Autodesk Inventor part; units mm, degrees
ref_plane "YZ Plane" through (0, 0, 0) normal (1, 0, 0) x (0, 1, 0)
ref_plane "XZ Plane" through (0, 0, 0) normal (0, 1, 0) x (-1, 0, 0)
ref_plane "XY Plane" through (0, 0, 0) normal (0, 0, 1) x (1, 0, 0)
sketch "Эскиз1" plane through (0, 0, 0) normal (0, 0, 1) x (1, 0, 0)
  line L0 (50, -27) -> (-50, -27)
  line L1 (-50, -27) -> (-50, 27)
  line L2 (-50, 27) -> (50, 27)
  line L3 (50, 27) -> (50, -27)
  line L4 (50, -27) -> (-50, 27) construction
  line L5 (-50, -27) -> (50, 27) construction
  circle A0 centre (27.5, 0) radius 16.1
  point P0 (0, 0)
  point P1 (0, 0)
  dimension "d0" = 100
  dimension "d1" = 54
  dimension "d2" = 32.2
  dimension "d3" = 22.5
extrude "Выдавливание1" add sketch "Эскиз1" along normal blind 10
sketch "Эскиз2" plane through (0, 0, 0) normal (0, 0, -1) x (-1, 0, 0)
  circle A0 centre (-27.5, 0) radius 16.1
  circle A1 centre (-27.5, 0) radius 14
  point P0 (0, 0)
  dimension "d6" = 28
extrude "Выдавливание2" add sketch "Эскиз2" against normal blind 3
sketch "Эскиз3" plane through (0, 0, 10) normal (0, 0, 1) x (1, 0, 0)
  line L0 (-5.5, -22) -> (-5.5, 22)
  circle A0 centre (-27.5, 0) radius 18.5
  line L1 (-27.5, -18.5) -> (-62.6366, -18.5)
  line L2 (-62.6366, -18.5) -> (-62.6366, 18.5)
  line L3 (-62.6366, 18.5) -> (-27.5, 18.5)
  point P0 (0, 0)
  dimension "d9" = 37
  dimension "d10" = 22
extrude "Выдавливание3" cut sketch "Эскиз3" against normal blind 28.4
sketch "Эскиз4" plane through (0, 0, 10) normal (0, 0, 1) x (1, 0, 0)
  line L0 (-5.5, -22) -> (-5.5, 22)
  line L1 (-51.5, 22) -> (-5.5, 22)
  line L2 (-5.5, 22) -> (-5.5, -22)
  line L3 (-5.5, -22) -> (-51.5, -22)
  line L4 (-51.5, -22) -> (-51.5, 22)
  line L5 (-51.5, 22) -> (-5.5, -22) construction
  line L6 (-5.5, 22) -> (-51.5, -22) construction
  point P0 (0, 0)
  point P1 (-28.5, 0)
  dimension "d13" = 46
  dimension "d14" = 44
extrude "Выдавливание4" cut sketch "Эскиз4" against normal blind 6
sketch "Эскиз6" plane through (-50, 27, 0) normal (0, 1, 0) x (1, 0, 0)
  circle A0 centre (95, -5) radius 1.25
  circle A1 centre (50, -5) radius 1.25
  circle A2 centre (5, -5) radius 1.25
  line L0 (100, 0) -> (100, -10)
  line L1 (0, 0) -> (0, -10)
  line L2 (0, 0) -> (100, 0)
  point P0 (50, 0)
  point P1 (100, -5)
  point P2 (50, 0)
  dimension "d22" = 2.5
  dimension "d23" = 2.5
  dimension "d24" = 2.5
  dimension "d25" = 5
  dimension "d26" = 5
extrude "Выдавливание6" cut sketch "Эскиз6" against normal up to surface (5 mm away)
sketch "Эскиз7" plane through (0, 0, 10) normal (0, 0, 1) x (1, 0, 0)
  circle A0 centre (27.5, 22.5) radius 1.25
  circle A1 centre (27.5, -22.5) radius 1.25
  circle A2 centre (27.5, 0) radius 16.1
  point P0 (27.5, 0)
  dimension "d40" = 2.5
  dimension "d41" = 2.5
  dimension "d42" = 22.5
  dimension "d43" = 22.5
extrude "Выдавливание7" cut sketch "Эскиз7" against normal blind 10 contours A0 | A1
chamfer "Фаска3" distance 2 angle 45 2 edges at (26.25, -22.5, 10) (26.25, 22.5, 10)
equation "\"d22\" = d23"
equation "\"d23\" = d24"
properties part number "крепление подшипникового блока левая часть"
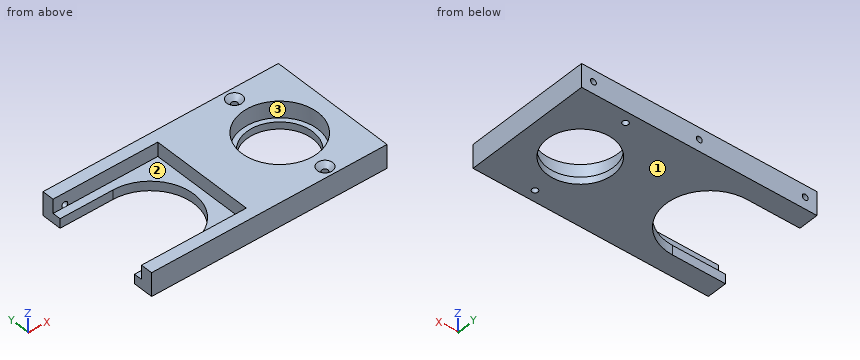
Part model, mm, in its own coordinate system. Face numbers are marked on the shaded views. A direction names the side the tool comes from. Coordinates: 2 decimals unless noted, no trailing zeros. Loops run counter-clockwise (first coordinate to the right, second up) from the corner with the lowest first, then second, coordinate; pieces in that order, holes last. Notation, with made-up numbers: M 4,64.25 L 23,64.25 A32 ccw 23,100.25 Z; hole C 34,81 d1. An arc over 180 degrees is marked long. Use a Markdown table: item, result. Add a question column.
Q1. Probe L1, parallel to Y at x = 27.5, z = 4.5; L2, parallel to X at y = 25.4, z = 5; L3, parallel to X at y = 0, z = 5.25. List the from-to ranges inside material, lowest first.
Q2. Pin check, flat tips, straight feed: P1, Ø3, axis at x = 27.5, y = 22.5, coming from the +Z side; P2, Ø1.5, axis at x = 45, z = 5, coming from the +Y side; P3, Ø5, axis at y = -3, z = 7, coming from the -X side. Stop position of each tip, or through.
Q3. Cut at B-B (x = -33.5). Write the cut outline in (y, z).
Q4. Cut at A-A (z = 5). Write the cut outline in (x, y).
Q5. Cut at D-D (x = 27.5). Write the cut outline in (y, z), and give its area (3 significant figures).
Q6. Cut at C-C (y = -5.5). Write the cut outline in (x, z).
Q7. Which spindle directions (+Z, -Z, +X, -X, +Y, -Y) get a long thin tool onto all of the face, cutting with end or side? Do the marked faces 1, 2 and 3. Say none if no direction does.
Worked out:
| question | item | result |
|---|---|---|
| 1 | L1 | y = -27 to -23.75, -21.25 to -16.1, 16.1 to 21.25, 23.75 to 27 |
| 1 | L2 | x = -50 to -46.25, -43.75 to -1.25, 1.25 to 43.75, 46.25 to 50 |
| 1 | L3 | x = -5.5 to 11.4, 43.6 to 50 |
| 2 | P1 | stops at z = 8.25 |
| 2 | P2 | stops at y = 22 |
| 2 | P3 | stops at x = -5.5 |
| 3 | outline | M -27,0 L -18.5,0 L -18.5,4 L -22,4 L -22,10 L -27,10 Z; M 18.5,0 L 27,0 L 27,10 L 22,10 L 22,4 L 18.5,4 Z |
| 4 | outline | M -50,-27 L 50,-27 L 50,27 L 46.25,27 L 46.25,22 L 43.75,22 L 43.75,27 L 1.25,27 L 1.25,22 L -1.25,22 L -1.25,27 L -43.75,27 L -43.75,22 L -5.5,22 L -5.5,-22 L -50,-22 Z; M -50,22 L -46.25,22 L -46.25,27 L -50,27 Z; hole C 27.5,0 d32.2; hole C 27.5,-22.5 d2.5; hole C 27.5,22.5 d2.5 |
| 5 | outline | M -27,0 L -23.75,0 L -23.75,8 L -25.75,10 L -27,10 Z; M -21.25,0 L -14,0 L -14,3 L -16.1,3 L -16.1,10 L -19.25,10 L -21.25,8 Z; M 14,0 L 21.25,0 L 21.25,8 L 19.25,10 L 16.1,10 L 16.1,3 L 14,3 Z; M 23.75,0 L 27,0 L 27,10 L 25.75,10 L 23.75,8 Z |
| 5 | area | 173 mm2 |
| 6 | outline | M -9.84,0 L 14.63,0 L 14.63,3 L 12.37,3 L 12.37,10 L -5.5,10 L -5.5,4 L -9.84,4 Z; M 40.37,0 L 50,0 L 50,10 L 42.63,10 L 42.63,3 L 40.37,3 Z |
| 7 | face 1 | -Z, +X, -X, +Y, -Y |
| 7 | face 2 | +Z, -X |
| 7 | face 3 | +Z |
